Verification items for the finished model (mm, model axes). Round coordinates to 2 decimals unless told otherwise and drop trailing zeros. Write each loop counter-clockwise with the first axis right and the second up, starting at its lowest first coordinate (ties: lowest second). Pieces come first, ordered by that corner, then holes. Notation, with made-up numbers: (52, 65) -> (84, 65) arc R4 ccw to (84, 71) -> close; hole circle Ø4 at (50.5, -35). An arc over 180 degrees is marked (long way). Answer as a JSON object with one key per item and string values. Group by question number.
(1) Gauge pin test, flat ends, axial feed: pin 1 Ø1.5 at (y, z) = (3, -3.5) entering from +X; pin 2 Ø2 at (y, z) = (1.5, -3.5) entering from +X. Record the tip position at first contact, or that the pin passes through.
(2) Scan lines: L1, parallel to X at y = 0.7, z = 0.25; L2, parallel to X at y = 1.9, z = -0.5; L3, parallel to X at y = 1.6, z = 2.25. Record each from-to range of solid material in increasing order. Write a range as from..to.
(3) Sectioned sample at A-A on z = 0. Record the cut outline in (x, y).
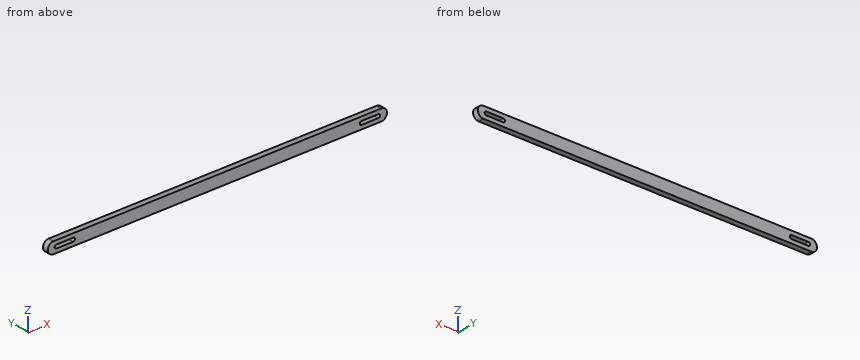
```python
from build123d import *

# Parameters (mm, degrees)
EXTRUDE_1_DEPTH = 5


with BuildPart() as part:
    # 草圖1 → 填料-伸長1 (new body)
    with BuildSketch(Plane(origin=(0, 0, 0), x_dir=(1, 0, 0), z_dir=(0, 1, 0))):
        with BuildLine():
            Line((-145.5, 5), (145.5, 5))
            ThreePointArc((145.5, 5), (150.5, 0), (145.5, -5))
            Line((145.5, -5), (-145.5, -5))
            ThreePointArc((-145.5, -5), (-150.5, 0), (-145.5, 5))
        make_face()
        with BuildLine():
            Line((-127.890062181, -1.55), (-142.830345758, -1.55))
            ThreePointArc((-142.830345758, -1.55), (-144.380345758, 0), (-142.830345758, 1.55))
            Line((-142.830345758, 1.55), (-127.890062181, 1.55))
            ThreePointArc((-127.890062181, 1.55), (-126.340062181, 0), (-127.890062181, -1.55))
        make_face(mode=Mode.SUBTRACT)
        with BuildLine():
            Line((127.890062181, -1.55), (142.830345758, -1.55))
            ThreePointArc((142.830345758, -1.55), (144.380345758, 0), (142.830345758, 1.55))
            Line((142.830345758, 1.55), (127.890062181, 1.55))
            ThreePointArc((127.890062181, 1.55), (126.340062181, 0), (127.890062181, -1.55))
        make_face(mode=Mode.SUBTRACT)
    extrude(amount=EXTRUDE_1_DEPTH)


solid = part.part
```
Computed values:
{
 "1": {"pin 1": "x = 149.68", "pin 2": "x = 149.83"},
 "2": {"L1": "-150.49..-144.36, -126.36..126.36, 144.36..150.49", "L2": "-150.47..-144.3, -126.42..126.42, 144.3..150.47", "L3": "-149.97..149.97"},
 "3": {"outline": "(-150.5, 0) -> (-144.38, 0) -> (-144.38, 5) -> (-150.5, 5) -> close; (-126.34, 0) -> (126.34, 0) -> (126.34, 5) -> (-126.34, 5) -> close; (144.38, 0) -> (150.5, 0) -> (150.5, 5) -> (144.38, 5) -> close"}
}
